Source: CAD feature listing. Evaluate the final solid. Frame: model axes, mm. Round coordinates to 2 decimals unless told otherwise and drop trailing zeros. Order: outer loops, then holes, each group sorted by start corner. A loop starts at its lowest first (then second) coordinate and runs counter-clockwise, first axis right, second up. Notation, with made-up numbers: (19, 20) -> (39, 20) arc R19 ccw to (39, 45) -> close; hole circle Ø3 at (85, -14.5). An arc over 180 degrees is marked (long way). Answer as CSV lines item,"result".
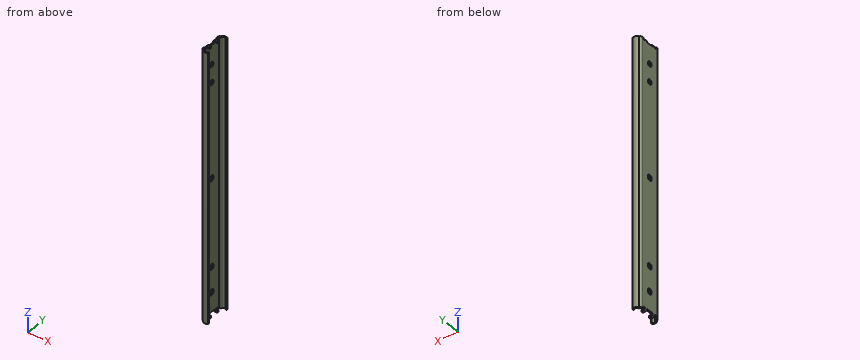
Autodesk Inventor part; units mm, degrees
ref_plane "to_retainer_XY" through (0, 0, 0) normal (0, 0, 1) x (1, 0, 0)
ref_plane "to_retainer_YZ" through (0, 0, 0) normal (1, 0, 0) x (0, 1, 0)
ref_plane "to_retainer_ZX" through (0, 0, 0) normal (0, 1, 0) x (0, 0, 1)
sketch "_____1" plane through (0, 0, 0) normal (0, 0, 1) x (1, 0, 0)
  line L0 (-2.85, 5.26) -> (-2.85, -5.26)
  arc A0 (-2.85, -5.26) -> (-2.0307, -6.4679) centre (-1.55, -5.26) ccw
  line L1 (-2.0307, -6.4679) -> (-1.8349, -6.5458)
  arc A1 (-1.8349, -6.5458) -> (1.43, -7.1482) centre (0, -5.75) ccw
  line L2 (1.43, -7.1482) -> (1.43, -6.5756)
  line L3 (1.43, -6.5756) -> (1.0392, -6.35)
  arc A2 (-1.1009, -6.2275) -> (1.0392, -6.35) centre (0, -5.75) ccw
  arc A3 (-1.1009, -6.2275) -> (-1.5391, -5.8025) centre (-1.8349, -6.5458) ccw
  line L4 (-1.5391, -5.8025) -> (-1.7349, -5.7246)
  arc A4 (-2.05, -5.26) -> (-1.7349, -5.7246) centre (-1.55, -5.26) ccw
  line L5 (-2.05, -5.26) -> (-2.05, 5.26)
  arc A5 (-1.7349, 5.7246) -> (-2.05, 5.26) centre (-1.55, 5.26) ccw
  line L6 (-1.7349, 5.7246) -> (-1.5391, 5.8025)
  arc A6 (-1.5391, 5.8025) -> (-1.1009, 6.2275) centre (-1.8349, 6.5458) ccw
  arc A7 (1.0392, 6.35) -> (-1.1009, 6.2275) centre (0, 5.75) ccw
  line L7 (1.0392, 6.35) -> (1.43, 6.5756)
  line L8 (1.43, 6.5756) -> (1.43, 7.1482)
  arc A8 (1.43, 7.1482) -> (-1.8349, 6.5458) centre (0, 5.75) ccw
  line L9 (-1.8349, 6.5458) -> (-2.0307, 6.4679)
  arc A9 (-2.0307, 6.4679) -> (-2.85, 5.26) centre (-1.55, 5.26) ccw
extrude "Extrusion1" add sketch "_____1" against normal blind 150
sketch "_____3" plane through (0, 0, 0) normal (0, 0, 1) x (1, 0, 0)
  line L0 (-2.05, 3.6) -> (-2.05, 2.2)
  line L1 (-2.05, 2.2) -> (-0.95, 2.2)
  arc A0 (-0.95, 2.2) -> (-0.45, 2.7) centre (-0.95, 2.7) ccw
  line L2 (-0.45, 2.7) -> (-0.45, 2.9484)
  arc A1 (-0.45, 2.9484) -> (-0.8206, 3.4314) centre (-0.95, 2.9484) ccw
  line L3 (-0.8206, 3.4314) -> (-1.45, 3.6)
  line L4 (-1.45, 3.6) -> (-2.05, 3.6)
extrude "Extrusion2" add sketch "_____3" against normal blind 0.8
sketch "_____5" plane through (0, 0, 0) normal (0, 0, 1) x (1, 0, 0)
  line L0 (-2.05, -3.6) -> (-1.45, -3.6)
  line L1 (-1.45, -3.6) -> (-0.8206, -3.4314)
  arc A0 (-0.8206, -3.4314) -> (-0.45, -2.9484) centre (-0.95, -2.9484) ccw
  line L2 (-0.45, -2.9484) -> (-0.45, -2.7)
  arc A1 (-0.45, -2.7) -> (-0.95, -2.2) centre (-0.95, -2.7) ccw
  line L3 (-0.95, -2.2) -> (-2.05, -2.2)
  line L4 (-2.05, -2.2) -> (-2.05, -3.6)
extrude "Extrusion3" add sketch "_____5" against normal blind 0.8
sketch "_____4" plane through (0, 0, 0) normal (1, 0, 0) x (0, 1, 0)
  line L0 (7.75, 1) -> (-7.75, 1)
  line L1 (-7.75, 1) -> (-7.75, 0)
  line L2 (-7.75, 0) -> (-4.9, 0)
  arc A0 (-4.6, -0.3) -> (-4.9, 0) centre (-4.9, -0.3) ccw
  line L3 (-4.6, -0.3) -> (-4.6, -0.7)
  arc A1 (-4.6, -0.7) -> (-4.1, -1.2) centre (-4.1, -0.7) ccw
  arc A2 (-4.1, -1.2) -> (-3.6, -0.7) centre (-4.1, -0.7) ccw
  line L4 (-3.6, -0.7) -> (-3.6, 0)
  line L5 (-3.6, 0) -> (-2.2, 0)
  line L6 (-2.2, 0) -> (-2.2, -0.7)
  arc A3 (-2.2, -0.7) -> (-1.7, -1.2) centre (-1.7, -0.7) ccw
  line L7 (-1.7, -1.2) -> (1.7, -1.2)
  arc A4 (1.7, -1.2) -> (2.2, -0.7) centre (1.7, -0.7) ccw
  line L8 (2.2, -0.7) -> (2.2, 0)
  line L9 (2.2, 0) -> (3.6, 0)
  line L10 (3.6, 0) -> (3.6, -0.7)
  arc A5 (3.6, -0.7) -> (4.1, -1.2) centre (4.1, -0.7) ccw
  arc A6 (4.1, -1.2) -> (4.6, -0.7) centre (4.1, -0.7) ccw
  line L11 (4.6, -0.7) -> (4.6, -0.3)
  arc A7 (4.9, 0) -> (4.6, -0.3) centre (4.9, -0.3) ccw
  line L12 (4.9, 0) -> (7.75, 0)
  line L13 (7.75, 0) -> (7.75, 1)
extrude "Extrusion4" cut sketch "_____4" against normal blind 4.28
sketch "_____6" plane through (0, 0, 0) normal (0, 1, 0) x (1, 0, 0)
  line L0 (-2.85, 0.8) -> (-2.85, 0)
  line L1 (-2.85, 0) -> (-2.05, 0)
  arc A0 (-2.85, 0.8) -> (-2.05, 0) centre (-2.05, 0.8) ccw
extrude "Extrusion5" cut sketch "_____6" along normal mid plane 8.2
sketch "_____2" plane through (0, 0, -150) normal (0, 0, 1) x (1, 0, 0)
  line L0 (-2.05, 3.6) -> (-2.05, 2.2)
  line L1 (-2.05, 2.2) -> (-0.95, 2.2)
  arc A0 (-0.95, 2.2) -> (-0.45, 2.7) centre (-0.95, 2.7) ccw
  line L2 (-0.45, 2.7) -> (-0.45, 2.9484)
  arc A1 (-0.45, 2.9484) -> (-0.8206, 3.4314) centre (-0.95, 2.9484) ccw
  line L3 (-0.8206, 3.4314) -> (-1.45, 3.6)
  line L4 (-1.45, 3.6) -> (-2.05, 3.6)
extrude "Extrusion6" add sketch "_____2" along normal blind 0.8
sketch "_____7" plane through (0, 0, -150) normal (0, 0, 1) x (1, 0, 0)
  line L0 (-2.05, -3.6) -> (-1.45, -3.6)
  line L1 (-1.45, -3.6) -> (-0.8206, -3.4314)
  arc A0 (-0.8206, -3.4314) -> (-0.45, -2.9484) centre (-0.95, -2.9484) ccw
  line L2 (-0.45, -2.9484) -> (-0.45, -2.7)
  arc A1 (-0.45, -2.7) -> (-0.95, -2.2) centre (-0.95, -2.7) ccw
  line L3 (-0.95, -2.2) -> (-2.05, -2.2)
  line L4 (-2.05, -2.2) -> (-2.05, -3.6)
extrude "Extrusion7" add sketch "_____7" along normal blind 0.8
sketch "_____8" plane through (-2.85, 0, 0) normal (1, 0, 0) x (0, 0, -1)
  arc A0 (148.8, -4.1) -> (149.3, -4.6) centre (149.3, -4.1) ccw
  line L0 (149.3, -4.6) -> (149.7, -4.6)
  arc A1 (150, -4.9) -> (149.7, -4.6) centre (149.7, -4.9) ccw
  line L1 (150, -4.9) -> (150, -7.75)
  line L2 (150, -7.75) -> (151, -7.75)
  line L3 (151, -7.75) -> (151, 7.75)
  line L4 (151, 7.75) -> (150, 7.75)
  line L5 (150, 7.75) -> (150, 4.9)
  arc A2 (149.7, 4.6) -> (150, 4.9) centre (149.7, 4.9) ccw
  line L6 (149.7, 4.6) -> (149.3, 4.6)
  arc A3 (149.3, 4.6) -> (148.8, 4.1) centre (149.3, 4.1) ccw
  arc A4 (148.8, 4.1) -> (149.3, 3.6) centre (149.3, 4.1) ccw
  line L7 (149.3, 3.6) -> (150, 3.6)
  line L8 (150, 3.6) -> (150, 2.2)
  line L9 (150, 2.2) -> (149.3, 2.2)
  arc A5 (149.3, 2.2) -> (148.8, 1.7) centre (149.3, 1.7) ccw
  line L10 (148.8, 1.7) -> (148.8, -1.7)
  arc A6 (148.8, -1.7) -> (149.3, -2.2) centre (149.3, -1.7) ccw
  line L11 (149.3, -2.2) -> (150, -2.2)
  line L12 (150, -2.2) -> (150, -3.6)
  line L13 (150, -3.6) -> (149.3, -3.6)
  arc A7 (149.3, -3.6) -> (148.8, -4.1) centre (149.3, -4.1) ccw
extrude "Extrusion8" cut sketch "_____8" along normal blind 0.8
sketch "_____9" plane through (0, 0, 0) normal (0, 1, 0) x (1, 0, 0)
  arc A0 (-2.05, 150) -> (-2.85, 149.2) centre (-2.05, 149.2) ccw
  line L0 (-2.05, 150) -> (-2.85, 150)
  line L1 (-2.85, 150) -> (-2.85, 149.2)
extrude "Extrusion9" cut sketch "_____9" along normal mid plane 8.2
sketch "Sketch10" plane through (-2.05, 5.26, 0) normal (1, 0, 0) x (0, 0, -1)
  point P0 (12, -5.26)
hole "Hole1" at (-2.05, 0, -12) direction (-1, 0, 0) diameter 2.8 depth 0.8
pattern_linear "Rectangular Pattern1" count 2 spacing 10 along (0, 0, -1) of "Hole1"
sketch "_____12" plane through (-2.85, 0, 0) normal (1, 0, 0) x (0, 0, -1)
  arc A0 (123.8, 1.4) -> (123.8, -1.4) centre (123.8, 0) ccw
  line L0 (123.8, -1.4) -> (124.2, -1.4)
  arc A1 (124.2, -1.4) -> (124.2, 1.4) centre (124.2, 0) ccw
  line L1 (124.2, 1.4) -> (123.8, 1.4)
extrude "Extrusion10" cut sketch "_____12" along normal blind 0.8
sketch "_____13" plane through (-2.85, 0, 0) normal (1, 0, 0) x (0, 0, -1)
  arc A0 (137.8, 1.4) -> (137.8, -1.4) centre (137.8, 0) ccw
  line L0 (137.8, -1.4) -> (138.2, -1.4)
  arc A1 (138.2, -1.4) -> (138.2, 1.4) centre (138.2, 0) ccw
  line L1 (138.2, 1.4) -> (137.8, 1.4)
extrude "Extrusion11" cut sketch "_____13" along normal blind 0.8
sketch "_____14" plane through (-2.85, 0, 0) normal (1, 0, 0) x (0, 0, -1)
  arc A0 (74.8, 1.4) -> (74.8, -1.4) centre (74.8, 0) ccw
  line L0 (74.8, -1.4) -> (75.2, -1.4)
  arc A1 (75.2, -1.4) -> (75.2, 1.4) centre (75.2, 0) ccw
  line L1 (75.2, 1.4) -> (74.8, 1.4)
extrude "Extrusion12" cut sketch "_____14" along normal blind 0.8
ref_plane "to_retainer_XY" through (0, 0, 0) normal (0, 0, 1) x (1, 0, 0)
ref_plane "to_retainer_YZ" through (0, 0, 0) normal (1, 0, 0) x (0, 1, 0)
ref_plane "to_retainer_ZX" through (0, 0, 0) normal (0, 1, 0) x (0, 0, 1)
properties part number "SSRC215_or" material "ステンレス鋼"
1. Pin query (flat end, axial travel): pin 1 (3 mm diameter, centred on y = -3.5, z = -117, fed in from +X); pin 2 (0.9 mm diameter, centred on x = -2.5, y = -0.5, fed in from -Z); pin 3 (2 mm diameter, centred on y = 0, z = -22, fed in from +X); pin 4 (0.6 mm diameter, centred on x = -2.5, z = -0.5, fed in from -Y). Return the tip coordinate at first contact, or that it passes through.
Results below:
pin 1,"x = -2.05"
pin 2,"z = -148.8"
pin 3,"through"
pin 4,"y = -6.39"
2. Section query B-B on z = -82. Return loops of the section in (x, y).
Results below:
outline,"(-2.85, -5.26) arc R1.3 ccw to (-2.03, -6.47) -> (-1.83, -6.55) arc R2 ccw to (1.43, -7.15) -> (1.43, -6.58) -> (1.04, -6.35) arc R1.2 cw to (-1.1, -6.23) arc R0.8 ccw to (-1.54, -5.8) -> (-1.73, -5.72) arc R0.5 cw to (-2.05, -5.26) -> (-2.05, 5.26) arc R0.5 cw to (-1.73, 5.72) -> (-1.54, 5.8) arc R0.8 ccw to (-1.1, 6.23) arc R1.2 cw to (1.04, 6.35) -> (1.43, 6.58) -> (1.43, 7.15) arc R2 ccw to (-1.83, 6.55) -> (-2.03, 6.47) arc R1.3 ccw to (-2.85, 5.26) -> close"
3. Line query: L1, parallel to Z at x = -2.3, y = 0; L2, parallel to Y at x = -2.25, z = -12; L3, parallel to Y at x = -2.4, z = -12. Output: solid intervals per line, ascending. Write a range as [from, to].
Results below:
L1,"[-148.8, -139.6], [-136.4, -125.6], [-122.4, -76.6], [-73.4, -23.4], [-20.6, -13.4], [-10.6, -1.2]"
L2,"[-6.36, -1.4], [1.4, 6.36]"
L3,"[-6.24, -1.4], [1.4, 6.24]"
4. Section query A-A on y = 0. Return loops of the section in (x, z).
Results below:
outline,"(-2.85, -148.8) -> (-2.05, -148.8) -> (-2.05, -139.6) -> (-2.85, -139.6) -> close; (-2.85, -136.4) -> (-2.05, -136.4) -> (-2.05, -125.6) -> (-2.85, -125.6) -> close; (-2.85, -122.4) -> (-2.05, -122.4) -> (-2.05, -76.6) -> (-2.85, -76.6) -> close; (-2.85, -73.4) -> (-2.05, -73.4) -> (-2.05, -23.4) -> (-2.85, -23.4) -> close; (-2.85, -20.6) -> (-2.05, -20.6) -> (-2.05, -13.4) -> (-2.85, -13.4) -> close; (-2.85, -10.6) -> (-2.05, -10.6) -> (-2.05, -1.2) -> (-2.85, -1.2) -> close"
